Input: part model. Units: mm. Frame: model coordinates. Face numbers are marked on the shaded views. Coordinates: 2 decimals unless noted, no trailing zeros. Loops run counter-clockwise (first coordinate to the right, second up) from the corner with the lowest first, then second, coordinate; pieces in that order, holes last.
Item 1: Section D-D on x = 129. Return loops of the section in (y, z), and give its area (3 significant figures).
Item 2: Contact query for flat-ended pins moving along their axis: P1, Ø10, axis at x = 313.5, z = 17.5, coming from the +Y side; P2, Ø8, axis at x = 166.5, y = 13, coming from the +Z side; P3, Ø3, axis at x = 296, y = 6, coming from the -Z side. Output: stop coordinate, or through.
Item 3: Ray query, line 1 along X through (y, z) = (16, -15); line 2 along Y through (x, z) = (185, 0.5); line 3 along Z through (x, y) = (261.5, 1). Return the intervals inside material, ascending.
Item 4: Pull-direction query (X, two-part tool) for the marked faces 1 and 2; classes: released by +X, released by -X, zero draft, split by the parting line, or undercut.
Item 5: Section C-C on x = 52. Return loops of the section in (y, z), and give its area (3 significant figures).
Item 6: Section A-A on z = 0. Return loops of the section in (x, y), and give its area (3 significant figures).
```python
from build123d import *

# Parameters (mm, degrees)
CHAMFER1_SIZE = 2.5


with BuildPart() as part:
    # Sketch1 → Revolve1 (revolve)
    with BuildSketch(Plane(origin=(0, 0, 0), x_dir=(1, 0, 0), z_dir=(0, 1, 0)), mode=Mode.PRIVATE) as revolve1_sk:
        Polygon((365, 0), (365, 22.5), (275, 22.5), (275, 20), (90, 20), (90, 22.5), (0, 22.5), (0, 0), align=None)
    revolve(revolve1_sk.sketch.rotate(Axis((-60.584183673, 0, 0), (1, 0, 0)), 180), axis=Axis((-60.584183673, 0, 0), (1, 0, 0)))

    # Chamfer1
    chamfer1_edges = [part.edges().sort_by_distance(p)[0] for p in [
        (0, 0, -22.5),
        (365, 0, -22.5),
    ]]
    chamfer(chamfer1_edges, length=CHAMFER1_SIZE)


solid = part.part
```
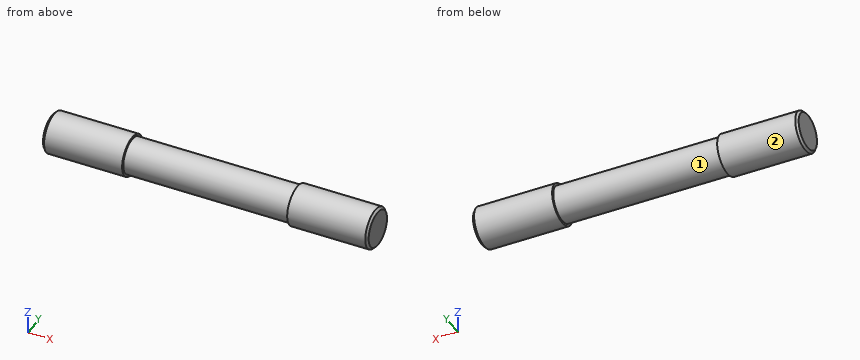
Results found:
1. outline: circle Ø40 at (0, 0)
1. area: 1,260 mm2
2. P1: stops at y = 18.71
2. P2: stops at z = 17.86
2. P3: stops at z = -22.05
3. line 1: x = 1.93 to 90, 275 to 363.07
3. line 2: y = -19.99 to 19.99
3. line 3: z = -19.97 to 19.97
4. face 1: undercut
4. face 2: zero draft
5. outline: circle Ø45 at (0, 0)
5. area: 1,590 mm2
6. outline: (0, -20) - (2.5, -22.5) - (90, -22.5) - (90, -20) - (275, -20) - (275, -22.5) - (362.5, -22.5) - (365, -20) - (365, 20) - (362.5, 22.5) - (275, 22.5) - (275, 20) - (90, 20) - (90, 22.5) - (2.5, 22.5) - (0, 20) - close
6. area: 15,500 mm2
